Solid Edge part; units mm, degrees
sketch "Sketch1" plane through (0, 0, 0) normal (0, 0, 1) x (1, 0, 0)
  line L0 (100, 0) -> (100, 40)
  line L1 (100, 40) -> (0, 40)
  line L2 (0, 40) -> (0, 0)
  line L3 (0, 0) -> (100, 0)
extrude "Protrusion1" add sketch "Sketch1" along normal blind 25
sketch "Sketch2" plane through (50, 0, 17.5) normal (0, -1, 0) x (1, 0, 0)
  circle A0 centre (-30, -10) radius 5
  circle A1 centre (0, -10) radius 5
  circle A2 centre (30, -10) radius 5
extrude "Cutout1" cut sketch "Sketch2" against normal up to next
hole "Hole_1" at (10, 10, 25) direction (0, 0, -1) diameter 3.3 depth 5
hole "Hole1" at (90, 10, 25) direction (0, 0, -1) diameter 3.3 depth 5
hole "Hole2" at (90, 30, 25) direction (0, 0, -1) diameter 3.3 depth 5
hole "Hole3" at (10, 30, 25) direction (0, 0, -1) diameter 3.3 depth 5
Read the model definition and answer for the solid it produces. Units are mm, in the model's axes. A direction names the side the tool comes from. Coordinates: 2 decimals unless noted, no trailing zeros. Write each loop counter-clockwise with the first axis right and the second up, starting at its lowest first coordinate (ties: lowest second). Pieces come first, ordered by that corner, then holes. Notation, with made-up numbers: (-7.5, -29.75) - (10.5, -29.75) arc R23 ccw to (10.5, 8.25) - close; hole circle Ø7 at (62, 46). An arc over 180 degrees is marked (long way). One line per question, with ' | ' between items.
Q1. This flat-tipped pin is pushed along its axis until it touches: P1, Ø2, axis at x = 10, y = 30, coming from the +Z side. Where does it stop, or does it pass through?
Result set:
P1: z = 20
Q2. Find section B-B, the plane y = 30. Write down the section's boundary in (x, z), plus the area to 3 significant figures.
Result set:
outline: (0, 0) - (100, 0) - (100, 25) - (91.65, 25) - (91.65, 20) - (88.35, 20) - (88.35, 25) - (11.65, 25) - (11.65, 20) - (8.35, 20) - (8.35, 25) - (0, 25) - close; hole circle Ø10 at (20, 7.5); hole circle Ø10 at (50, 7.5); hole circle Ø10 at (80, 7.5) | area: 2,230 mm^2
Q3. Find section D-D, the plane x = 10. Write down the section's boundary in (y, z).
Result set:
outline: (0, 0) - (40, 0) - (40, 25) - (31.65, 25) - (31.65, 20) - (28.35, 20) - (28.35, 25) - (11.65, 25) - (11.65, 20) - (8.35, 20) - (8.35, 25) - (0, 25) - close
Q4. Consider L1, parallel to X at y = 30, z = 21.7; L2, parallel to Y at x = 10, z = 22.65; L3, parallel to X at y = 7, z = 8.25. Determine where each line is inside the solid, lowest interval first. Write a range as [from, to].
Result set:
L1: [0, 8.35], [11.65, 88.35], [91.65, 100] | L2: [0, 8.35], [11.65, 28.35], [31.65, 40] | L3: [0, 15.06], [24.94, 45.06], [54.94, 75.06], [84.94, 100]
Q5. Find section A-A, the plane x = 80. Write down the section's boundary in (y, z), plus the area to 3 significant figures.
Result set:
outline: (0, 0) - (40, 0) - (40, 2.5) - (0, 2.5) - close; (0, 12.5) - (40, 12.5) - (40, 25) - (0, 25) - close | area: 600 mm^2
Q6. Find section C-C, the plane z = 6.25. Write down the section's boundary in (x, y), plus the area to 3 significant figures.
Result set:
outline: (0, 0) - (15.16, 0) - (15.16, 40) - (0, 40) - close; (24.84, 0) - (45.16, 0) - (45.16, 40) - (24.84, 40) - close; (54.84, 0) - (75.16, 0) - (75.16, 40) - (54.84, 40) - close; (84.84, 0) - (100, 0) - (100, 40) - (84.84, 40) - close | area: 2,840 mm^2
Q7. Determine the mould class of faces 1 (the flat face through (51, 40, 15)), 2 (the flat face through (90, 30, 20)), 3 (the flat face through (100, 20, 12)) for opening direction Y: +Y half, -Y half, draft (parallel to the pull), parting line (faces both ways), or undercut.
Result set:
face 1: +Y half | face 2: undercut | face 3: draft
Q8. For faces 4 (the cylindrical face through (11, 31.31, 22.46)), 5 (the cylindrical face through (19.349, 19.72, 12.457)), determine the directions among +Z, -Z, +X, -X, +Y, -Y from which every point of the face is accessible in a straight line to the end or side of a thin tool.
Result set:
face 4: +Z | face 5: +Y, -Y
